```python
from build123d import *

# Parameters (mm, degrees)
SKETCH1_R                = 2.159
SKETCH1_R_2              = 28.5115
BOSS_EXTRUDE1_DEPTH      = 9.525
SKETCH1_4_R              = 28.5115
SKETCH1_4_R_2            = 23.8125
FLUSH_BEZEL_DEPTH        = 9.525
SKETCH1_5_R              = 28.5115
SKETCH1_5_R_2            = 23.8125
BOSS_EXTRUDE4_DEPTH      = 6.35
SKETCH2_R                = 25.3365
CUT_EXTRUDE1_DEPTH       = 7.35
CUT_EXTRUDE1_DEPTH_BACK  = 9.525
SKETCH3_R                = 28.5115
CUT_EXTRUDE2_DEPTH       = 7.35
SKETCH4_R                = 25.3365
SKETCH4_R_2              = 23.8125
BOSS_EXTRUDE7_DEPTH      = 1.5875
M6_CLEARANCE_HOLE1_D     = 7
M6_CLEARANCE_HOLE1_DEPTH = 9.525
BOSS_EXTRUDE8_REACH      = 11.525
SKETCH8_R                = 25.3365
SKETCH8_R_2              = 23.8125
CUT_EXTRUDE3_DEPTH       = 6.35
BOSS_EXTRUDE9_DEPTH      = 9.525


with BuildPart() as part:
    # Sketch1 → Boss-Extrude1 (new body)
    with BuildSketch(Plane.XY):
        with BuildLine():
            Line((-26.9875, 30.1625), (26.9875, 30.1625))
            ThreePointArc((26.9875, 30.1625), (29.23256403, 29.23256403), (30.1625, 26.9875))
            Line((30.1625, 26.9875), (30.1625, -26.9875))
            ThreePointArc((30.1625, -26.9875), (29.23256403, -29.23256403), (26.9875, -30.1625))
            Line((26.9875, -30.1625), (-26.9875, -30.1625))
            ThreePointArc((-26.9875, -30.1625), (-29.23256403, -29.23256403), (-30.1625, -26.9875))
            Line((-30.1625, -26.9875), (-30.1625, 26.9875))
            ThreePointArc((-30.1625, 26.9875), (-29.23256403, 29.23256403), (-26.9875, 30.1625))
        make_face()
        with Locations((-26.9748, 26.9748)):
            Circle(SKETCH1_R, mode=Mode.SUBTRACT)
        with Locations((26.9748, 26.9748)):
            Circle(SKETCH1_R, mode=Mode.SUBTRACT)
        with Locations((26.9748, -26.9748)):
            Circle(SKETCH1_R, mode=Mode.SUBTRACT)
        Circle(SKETCH1_R_2, mode=Mode.SUBTRACT)
    extrude(amount=BOSS_EXTRUDE1_DEPTH)

    # Sketch1_4 → Flush Bezel (add)
    with BuildSketch(Plane.XY):
        Circle(SKETCH1_4_R)
        Circle(SKETCH1_4_R_2, mode=Mode.SUBTRACT)
    extrude(amount=FLUSH_BEZEL_DEPTH)

    # Sketch1_5 → Boss-Extrude4 (add)
    with BuildSketch(Plane.XY):
        Circle(SKETCH1_5_R)
        Circle(SKETCH1_5_R_2, mode=Mode.SUBTRACT)
    extrude(amount=-BOSS_EXTRUDE4_DEPTH)

    # Sketch2 → Cut-Extrude1 (cut, two sides)
    with BuildSketch(Plane(origin=(0, 0, 0), x_dir=(-1, 0, 0), z_dir=(0, 0, -1))) as cut_extrude1_sk:
        Circle(SKETCH2_R)
    extrude(amount=CUT_EXTRUDE1_DEPTH, mode=Mode.SUBTRACT)
    extrude(cut_extrude1_sk.sketch, amount=-CUT_EXTRUDE1_DEPTH_BACK, mode=Mode.SUBTRACT)

    # Sketch3 → Cut-Extrude2 (cut, through all)
    with BuildSketch(Plane(origin=(0, 0, 0), x_dir=(-1, 0, 0), z_dir=(0, 0, -1))):
        Circle(SKETCH3_R)
    extrude(amount=CUT_EXTRUDE2_DEPTH, mode=Mode.SUBTRACT)

    # Sketch4 → Boss-Extrude7 (add)
    with BuildSketch(Plane.XY.offset(9.525)):
        Circle(SKETCH4_R)
        Circle(SKETCH4_R_2, mode=Mode.SUBTRACT)
    extrude(amount=-BOSS_EXTRUDE7_DEPTH)

    # M6 Clearance Hole1
    with Locations(Plane.XY.offset(9.525)):
        with Locations((-22.45595798, -21.4503)):
            Hole(M6_CLEARANCE_HOLE1_D / 2, depth=M6_CLEARANCE_HOLE1_DEPTH)

    # Sketch8 → Boss-Extrude8 (add, up to next)
    with BuildSketch(Plane(origin=(0, 0, 0), x_dir=(-1, 0, 0), z_dir=(0, 0, -1)), mode=Mode.PRIVATE) as boss_extrude8_sk1:
        Circle(SKETCH8_R)
        Circle(SKETCH8_R_2, mode=Mode.SUBTRACT)
    boss_extrude8_tool1 = extrude(boss_extrude8_sk1.sketch, amount=-BOSS_EXTRUDE8_REACH, mode=Mode.PRIVATE) - part.part
    add(boss_extrude8_tool1.solids().sort_by_distance((24.619876, 0, 0))[0])

    # Sketch9 → Cut-Extrude3 (cut)
    with BuildSketch(Plane(origin=(0, 0, 0), x_dir=(-1, 0, 0), z_dir=(0, 0, -1))):
        Polygon((25.823554026, -36.043216197), (37.048874177, -24.817896045), (19.088361935, -6.857383803), (7.863041784, -18.082703955), align=None)
    extrude(amount=-CUT_EXTRUDE3_DEPTH, mode=Mode.SUBTRACT)

    # Sketch10 → Boss-Extrude9 (add)
    with BuildSketch(Plane.XY.offset(9.525)):
        with BuildLine():
            Line((26.9875, 31.75), (-26.9875, 31.75))
            ThreePointArc((-26.9875, 31.75), (-30.355096045, 30.355096045), (-31.75, 26.9875))
            Line((-31.75, 26.9875), (-31.75, -26.9875))
            ThreePointArc((-31.75, -26.9875), (-30.355096045, -30.355096045), (-26.9875, -31.75))
            Line((-26.9875, -31.75), (26.9875, -31.75))
            ThreePointArc((26.9875, -31.75), (30.355096045, -30.355096045), (31.75, -26.9875))
            Line((31.75, -26.9875), (31.75, 26.9875))
            ThreePointArc((31.75, 26.9875), (30.355096045, 30.355096045), (26.9875, 31.75))
        make_face()
        with BuildLine():
            Line((26.9875, 30.1625), (-26.9875, 30.1625))
            ThreePointArc((-26.9875, 30.1625), (-29.23256403, 29.23256403), (-30.1625, 26.9875))
            Line((-30.1625, 26.9875), (-30.1625, -26.9875))
            ThreePointArc((-30.1625, -26.9875), (-29.23256403, -29.23256403), (-26.9875, -30.1625))
            Line((-26.9875, -30.1625), (26.9875, -30.1625))
            ThreePointArc((26.9875, -30.1625), (29.23256403, -29.23256403), (30.1625, -26.9875))
            Line((30.1625, -26.9875), (30.1625, 26.9875))
            ThreePointArc((30.1625, 26.9875), (29.23256403, 29.23256403), (26.9875, 30.1625))
        make_face(mode=Mode.SUBTRACT)
    extrude(amount=-BOSS_EXTRUDE9_DEPTH)


solid = part.part
```
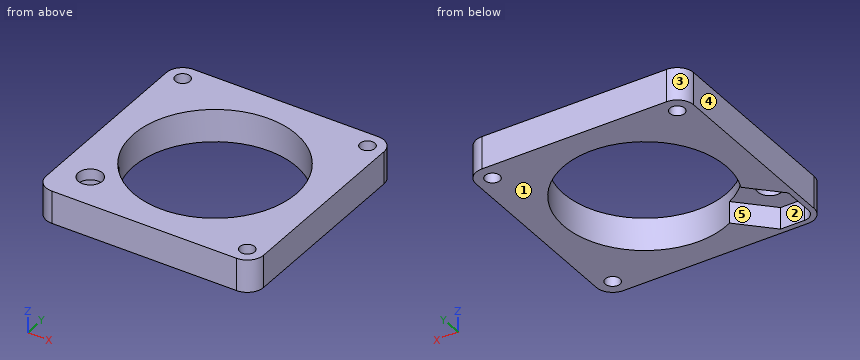
Geometry: final body of the model. Coordinates: model frame, mm. Face numbers are marked on the shaded views. A direction names the side the tool comes from. Round coordinates to 2 decimals unless told otherwise and drop trailing zeros. Write each loop counter-clockwise with the first axis right and the second up, starting at its lowest first coordinate (ties: lowest second). Pieces come first, ordered by that corner, then holes. Notation, with made-up numbers: M 66,75 L 91,75 A12 ccw 91,81 Z; hole C 38.25,83.25 d3. An arc over 180 degrees is marked long. Answer in a Markdown table with one row per item. Add a question column.
(1) Contact query for a flat-ended pin moving along its axis: pin 1 (4 mm diameter, centred on x = -26.97, y = 26.97, fed in from -Z). Output: stop coordinate, or through.
(2) Ray query, L1, parallel to X at y = 0.5, z = 1; L2, parallel to Y at x = 25, z = 3.75. Return the intervals inside material, ascending.
(3) Draft query along Y for the marked faces 3, 4 and 5. Return one class per face: pulls with the +Y half, pulls with the -Y half, needs draft (parallel to the pull), parting line crosses it, or undercut.
(4) Cut plane D-D, the plane y = -16.5. Return the cut outline in (x, z) (3 decimals), then the cut area to 3 significant figures.
(5) Reachability of the marked faces 1 and 2 from +Z, -Z, +X, -X, +Y, -Y: full face, straight path, thin tool, end or side. Return the list, or none.
(6) Cut plane C-C, the plane z = 1.5. Give the number of separate pieces and of enclosed holes in the cut face, then the cut area to 3 significant figures.
Established:
| question | item | result |
|---|---|---|
| 1 | pin 1 | through |
| 2 | L1 | -31.75 to -23.81, 23.81 to 31.75 |
| 2 | L2 | -31.75 to -27.85, -26.1 to 26.1, 27.85 to 31.75 |
| 3 | face 3 | pulls with the +Y half |
| 3 | face 4 | needs draft |
| 3 | face 5 | undercut |
| 4 | outline | M -31.75,0 L -28.731,0 L -28.731,6.35 L -17.169,6.35 L -17.169,9.525 L -31.75,9.525 Z; M 17.169,0 L 31.75,0 L 31.75,9.525 L 17.169,9.525 Z |
| 4 | area | 204 mm² |
| 5 | face 1 | -Z, +X, -X, +Y, -Y |
| 5 | face 2 | -Z |
| 6 | separate pieces | 1 |
| 6 | enclosed holes | 4 |
| 6 | area | 1,950 mm² |
